Geometry: see drawing. Coordinates: mm, zero at the bounding-box minimum. A direction names the side the tool comes from. Give positions to 0.01 mm unless a question says otherwise; leave off trailing zeros. Loops run counter-clockwise (first coordinate to the right, second up) from the corner with the lowest first, then second, coordinate; pieces in that order, holes last. Notation, with made-up numbers: M 42.5,70 L 71.5,70 A21 ccw 71.5,85 Z; hole C 49.5,-5 d11. An arc over 180 degrees is marked long. Put each result on its own line as item: value.
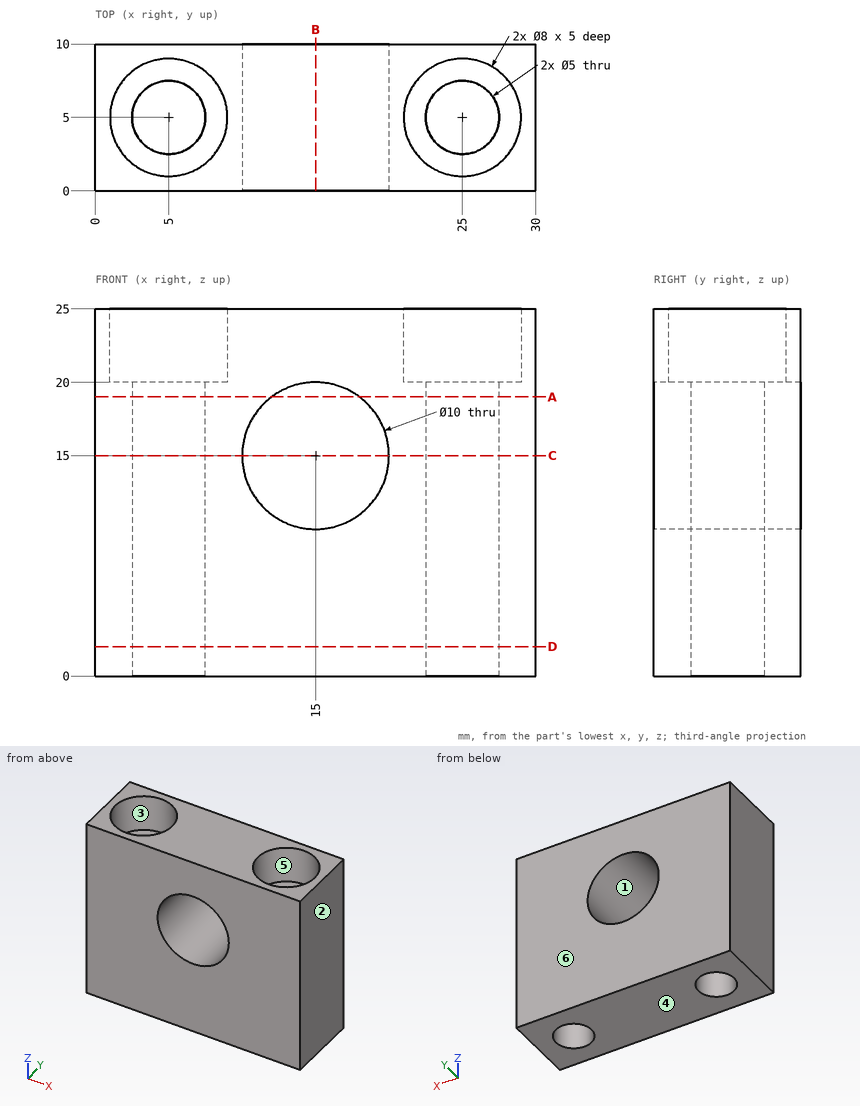
Item 1: Section A-A on z = 19. Output: boundary loops of the cut face in (x, y), then the cut area to 3 significant figures.
Output values:
outline: M 0,0 L 12,0 L 12,10 L 0,10 Z; M 18,0 L 30,0 L 30,10 L 18,10 Z; hole C 5,5 d5; hole C 25,5 d5
area: 201 mm²
Item 2: Mould query, pull axis X, two halves, no side actions, for the marked faces 1, 2, 3 and 4. Classes: pulls with the +X half, pulls with the -X half, needs draft (parallel to the pull), parting line crosses it, or undercut.
Output values:
face 1: undercut
face 2: pulls with the +X half
face 3: undercut
face 4: needs draft
Item 3: Line query: probe 1 along X at (y, z) = (5, 8.75); probe 2 along Z at (x, y) = (15, 2.75); probe 3 along Y at (x, z) = (5, 15.5). Output: solid intervals per line, ascending. Write a range as [from, to].
Output values:
probe 1: [0, 2.5], [7.5, 22.5], [27.5, 30]
probe 2: [0, 10], [20, 25]
probe 3: [0, 2.5], [7.5, 10]
Item 4: Section B-B on x = 15. Output: boundary loops of the cut face in (y, z).
Output values:
outline: M 0,0 L 10,0 L 10,10 L 0,10 Z; M 0,20 L 10,20 L 10,25 L 0,25 Z
Item 5: Pin query (flat end, axial travel): pin 1 Ø2.5 at (x, y) = (25.5, 6.5) entering from +Z. Return the tip coordinate at first contact, or that it passes through.
Output values:
pin 1: z = 20
Item 6: Section C-C on z = 15. Output: boundary loops of the cut face in (x, y).
Output values:
outline: M 0,0 L 10,0 L 10,10 L 0,10 Z; M 20,0 L 30,0 L 30,10 L 20,10 Z; hole C 5,5 d5; hole C 25,5 d5
Item 7: Section D-D on z = 2. Output: boundary loops of the cut face in (x, y).
Output values:
outline: M 0,0 L 30,0 L 30,10 L 0,10 Z; hole C 5,5 d5; hole C 25,5 d5
Item 8: Set-up query: the marked faces 5 and 6. Return all of +Z, -Z, +X, -X, +Y, -Y with unobstructed straight access to the full face (end or side cutting, diameter ignored); none if empty.
Output values:
face 5: +Z
face 6: +Z, -Z, +X, -X, +Y
